Input: part model. Units: mm. Frame: model coordinates. Face numbers are marked on the shaded views. A direction names the side the tool comes from. Coordinates: 2 decimals unless noted, no trailing zeros. Write each loop counter-clockwise with the first axis right and the second up, starting at its lowest first coordinate (ties: lowest second). Pieces come first, ordered by that corner, then holes. Notation, with made-up numbers: (14, 75) - (18, 75) arc R31 cw to (18, 99) - close; hole circle Ø7 at (66.5, 19.25). An arc over 180 degrees is marked (long way). One line per question, with ' | ' between items. Start each with the question number.
1) Reachability of the marked faces 1 and 2 from +Z, -Z, +X, -X, +Y, -Y: full face, straight path, thin tool, end or side. Return the list, or none.
2) Section query B-B on y = -174. Return loops of the section in (x, z) (3 decimals).
3) Section query C-C on z = 17. Return loops of the section in (x, y) (3 decimals).
4) First-contact query: P1, Ø12, axis at y = -56.5, z = 19, coming from the +X side (3 decimals); P2, Ø3, axis at x = -11.11, y = -219.08, coming from the -Z side; P3, Ø8, axis at x = -12.5, y = -218, coming from the +Z side (3 decimals). Flat tips, straight axial feed; report the tip coordinate or a pass-through.
5) Line query: line 1 (Y direction, x = -10.5, z = 1.25); line 2 (X direction, y = -18, z = 12.5) (3 decimals); line 3 (Z direction, x = -5.75, y = -102.5) (3 decimals). Output: solid intervals per line, ascending.
6) Section query A-A on y = -19.05. Return loops of the section in (x, z) (3 decimals).
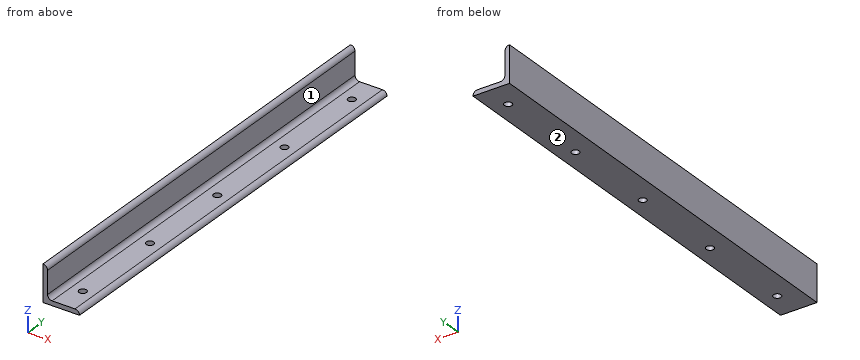
```python
from build123d import *

# Parameters (mm, degrees)
F1_DEPTH = 304.8
F2_R     = 2.6162
F3_DEPTH = 3.176


with BuildPart() as f1:
    # F0 (on Front) → F1 (new body)
    with BuildSketch(Plane.XZ):
        with BuildLine():
            Line((-25.4, 0), (0, 0))
            ThreePointArc((0, 0), (-0.929936, 2.245064), (-3.175, 3.175))
            Line((-3.175, 3.175), (-19.05, 3.175))
            ThreePointArc((-19.05, 3.175), (-21.295064, 4.104936), (-22.225, 6.35))
            Line((-22.225, 6.35), (-22.225, 22.225))
            ThreePointArc((-22.225, 22.225), (-23.154936, 24.470064), (-25.4, 25.4))
            Line((-25.4, 25.4), (-25.4, 0))
        make_face()
    extrude(amount=F1_DEPTH)

    # F2 (on face) → F3 (cut, through all)
    with BuildSketch(Plane.XY.offset(3.175)):
        with Locations((-11.1125, -285.75)):
            Circle(F2_R)
        with Locations((-11.1125, -19.05)):
            Circle(F2_R)
        with Locations((-11.1125, -219.075)):
            Circle(F2_R)
        with Locations((-11.1125, -152.4)):
            Circle(F2_R)
        with Locations((-11.1125, -85.725)):
            Circle(F2_R)
    extrude(amount=-F3_DEPTH, mode=Mode.SUBTRACT)


solid = f1.part
```
Answer key:
1) face 1: +Z, +X, +Y, -Y | face 2: -Z, +X, -X, +Y, -Y
2) outline: (-25.4, 0) - (0, 0) arc R3.175 ccw to (-3.175, 3.175) - (-19.05, 3.175) arc R3.175 cw to (-22.225, 6.35) - (-22.225, 22.225) arc R3.175 ccw to (-25.4, 25.4) - close
3) outline: (-25.4, -304.8) - (-22.225, -304.8) - (-22.225, 0) - (-25.4, 0) - close
4) P1: x = -22.225 | P2: through | P3: z = 3.175
5) line 1: -304.8 to -288.29, -283.21 to -221.62, -216.53 to -154.94, -149.86 to -88.27, -83.18 to -21.59, -16.51 to 0 | line 2: -25.4 to -22.225 | line 3: 0 to 3.175
6) outline: (-25.4, 0) - (-13.729, 0) - (-13.729, 3.175) - (-19.05, 3.175) arc R3.175 cw to (-22.225, 6.35) - (-22.225, 22.225) arc R3.175 ccw to (-25.4, 25.4) - close; (-8.496, 0) - (0, 0) arc R3.175 ccw to (-3.175, 3.175) - (-8.496, 3.175) - close
